Part model, mm, in its own coordinate system. Face numbers are marked on the shaded views. A direction names the side the tool comes from. Coordinates: 2 decimals unless noted, no trailing zeros. Write each loop counter-clockwise with the first axis right and the second up, starting at its lowest first coordinate (ties: lowest second). Pieces come first, ordered by that corner, then holes. Notation, with made-up numbers: (58, -39) -> (86, -39) arc R11 cw to (86, -23) -> close; hole circle Ø6 at (59.5, 28.25). An arc over 180 degrees is marked (long way). Write item = value, one per line. Start each with the question number.
Q1. Tool access for the marked faces 1, 2 and 3: list every direction of +Z, -Z, +X, -X, +Y, -Y with a clear straight run to the whole face (end or side of a thin tool).
Q2. Band-saw the part on A-A, the plane z = 0. List the corners of the cut face in (x, y), plus the area to 3 significant figures.
Q3. Band-saw the part on B-B, the plane y = 16.25. List the corners of the cut face in (x, z), plus the area to 3 significant figures.
Q4. Band-saw the part on C-C, the plane y = 8.5. List the corners of the cut face in (x, z), plus the area to 3 significant figures.
Q5. Probe line 1 (Z direction, x = 0, y = 2.45); line 2 (Z direction, x = -1, y = 4.25); line 3 (Z direction, x = 6.5, y = 13). List the from-to ranges inside material, lowest first.
Q6. Pull direction X, two halves, no side cores. Call the marked faces 4, 5 and 6: released by +X, released by -X, zero draft, split by the parting line, or undercut.
Q7. Pin check, flat tips, straight feed: P1, Ø6, axis at x = 20, z = 18.5, coming from the -Y side; P2, Ø1.8, axis at x = -8.5, z = 3.5, coming from the +Y side; P3, Ø5.5, axis at y = 11, z = -7.5, coming from the -X side; P4, Ø4, axis at x = 0.5, y = 17, coming from the -Z side. Stop position of each tip, or through.
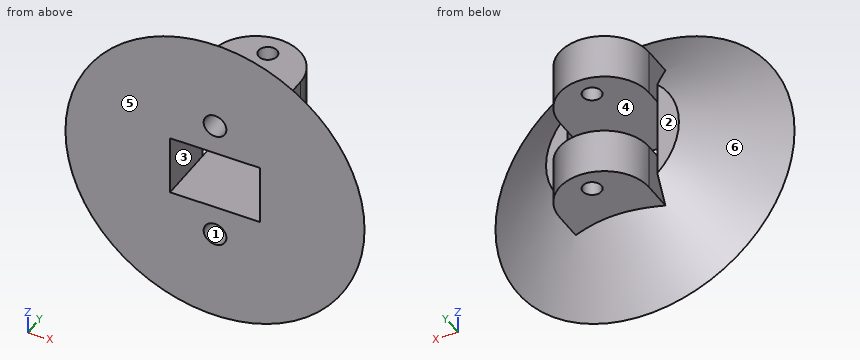
Autodesk Inventor part; units mm, degrees
ref_plane "РабПлоскость1" through (0, 10, 0) normal (0, -1, 0) x (1, 0, 0)
ref_plane "YZ Plane" through (0, 0, 0) normal (1, 0, 0) x (0, 1, 0)
ref_plane "XZ Plane" through (0, 0, 0) normal (0, 1, 0) x (-1, 0, 0)
sketch "Эскиз1" plane through (0, 0, 0) normal (0, 0, 1) x (1, 0, 0)
  line L0 (0, 0) -> (25, 0)
  line L1 (0, 0) -> (0, 18)
  line L2 (0, 18) -> (25, 0)
  line L3 (0, -3.6) -> (0, 21.6)
  dimension "d0" = 25
  dimension "d2" = 18
revolve "Вращение1" add sketch "Эскиз1" angle 360 about axis through (0, -10, 0) along (0, 1, 0)
ref_plane "РабПлоскость1" through (0, 10, 0) normal (0, -1, 0) x (1, 0, 0)
sketch "Эскиз2" plane through (0, 10, 0) normal (0, -1, 0) x (1, 0, 0)
  circle A0 centre (0, 0) radius 11.1111
extrude "Выдавливание1" cut sketch "Эскиз2" against normal blind 10
sketch "Эскиз3" plane through (0, 0, 0) normal (0, 0, 1) x (1, 0, 0)
  line L0 (-7.5, 12.5) -> (-7.5, 0)
  line L1 (-7.5, 0) -> (7.5, 0)
  line L2 (7.5, 0) -> (7.5, 12.5)
  arc A0 (7.5, 12.5) -> (-7.5, 12.5) centre (0, 12.5) ccw
  line L3 (0, 12.5) -> (0, 20) construction
  circle A1 centre (0, 16.25) radius 1.55
  point P0 (0, 0)
  point P1 (0, 0)
  dimension "d10" = 3.1
extrude "Выдавливание2" add sketch "Эскиз3" along normal mid plane 25
extrude "Выдавливание3" cut sketch "Эскиз3" along normal mid plane 10
sketch "Эскиз6" plane through (0, 0, 0) normal (0, -1, 0) x (1, 0, 0)
  circle A0 centre (-58.3547, -41.682) radius 1.575 construction
  circle A1 centre (-58.3429, -21.682) radius 1.575 construction
  circle A2 centre (-58.3547, -41.682) radius 1.35
  circle A3 centre (-58.3429, -21.682) radius 1.35
  point P0 (0, 0)
  dimension "d24" = 2.7
  dimension "d25" = 2.7
sketch "Эскиз7" plane through (0, 0, 0) normal (0, -1, 0) x (1, 0, 0)
  circle A0 centre (0, -10) radius 1.9
  circle A1 centre (0, 10) radius 1.9
  circle A2 centre (0, 0) radius 25
  line L0 (0, -10) -> (0, 10) construction
  dimension "d29" = 3.8
  dimension "d30" = 20
extrude "Выдавливание7" cut sketch "Эскиз7" against normal blind 5 contours A0 | A1
sketch "Эскиз8" plane through (0, 5, 10) normal (0, -1, 0) x (1, 0, 0)
  circle A0 centre (0, 0) radius 1.9
  circle A1 centre (0, -20) radius 1.9
  circle A2 centre (0, 0) radius 1.9
  circle A3 centre (0, 0) radius 1.65
  circle A4 centre (0, -20) radius 1.65
  point P0 (0, -10)
  dimension "d33" = 3.3
extrude "Выдавливание8" cut sketch "Эскиз8" against normal blind 5 contours A3 | A4
properties part number "стенд"
Ans:
q1.face_1 = -Y
q1.face_2 = +Z, -Z, -X, +Y
q1.face_3 = +Y, -Y
q2.outline = (-25, 0) -> (-7.5, 0) -> (-7.5, 10) -> (-11.11, 10) -> close; (7.5, 0) -> (25, 0) -> (11.11, 10) -> (7.5, 10) -> close
q2.area = 211 mm2
q3.outline = (-6.5, -12.5) -> (-1.55, -12.5) -> (-1.55, -5) -> (-6.5, -5) -> close; (-6.5, 5) -> (-1.55, 5) -> (-1.55, 12.5) -> (-6.5, 12.5) -> close; (1.55, -12.5) -> (6.5, -12.5) -> (6.5, -5) -> (1.55, -5) -> close; (1.55, 5) -> (6.5, 5) -> (6.5, 12.5) -> (1.55, 12.5) -> close
q3.area = 148 mm2
q4.outline = (-7.5, -12.5) -> (-4.22, -12.5) arc R13.19 ccw to (4.22, -12.5) -> (7.5, -12.5) -> (7.5, -10.86) arc R13.19 ccw to (7.5, 10.86) -> (7.5, 12.5) -> (4.22, 12.5) arc R13.19 ccw to (-4.22, 12.5) -> (-7.5, 12.5) -> (-7.5, 10.86) arc R13.19 ccw to (-7.5, -10.86) -> close; hole (-7.5, -5) -> (7.5, -5) -> (7.5, 5) -> (-7.5, 5) -> close; hole circle Ø3.3 at (0, -10); hole circle Ø3.3 at (0, 10)
q4.area = 389 mm2
q5.line_1 = -21.6 to -11.9, -8.1 to -5, 5 to 8.1, 11.9 to 21.6
q5.line_2 = -19.07 to -11.62, -8.38 to -5, 5 to 8.38, 11.62 to 19.07
q5.line_3 = -12.5 to -5, 5 to 12.5
q6.face_4 = undercut
q6.face_5 = zero draft
q6.face_6 = split by the parting line
q7.P1 = 0
q7.P2 = 10
q7.P3 = -11.58
q7.P4 = -12.5
